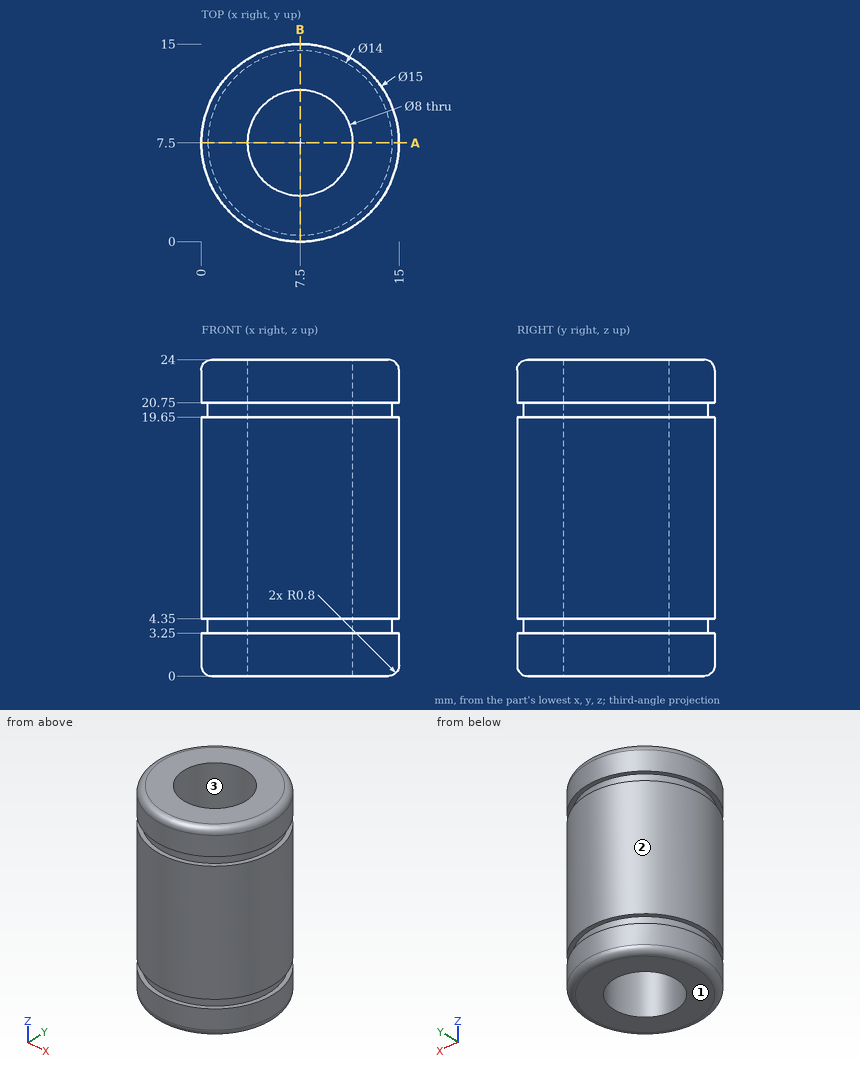
Geometry check sheet. Reference: drawing and pictorial views, mm from the part's lowest x, y, z. Coordinates: 2 decimals unless noted, no trailing zeros. Order: outer loops, then holes, each group sorted by start corner. A loop starts at its lowest first (then second) coordinate and runs counter-clockwise, first axis right, second up. Notation, with made-up numbers: (32, -13.5) - (72, -13.5) arc R24 cw to (72, 21.5) - close; hole circle Ø6 at (45, 41.25). An arc over 180 degrees is marked (long way). Answer in a Markdown table with one row per item. Add a question column.
1) Material ranges on line 1 along Y through (x, z) = (7.5, 16.25); line 2 along Z through (x, y) = (3.5, 1.5); line 3 along X through (y, z) = (5, 6.75), recorded low to high. Write a range as [from, to].
2) Cross-section at A-A, the plane y = 7.5. Record the cut outline in (x, z).
3) Gauge pin test, flat ends, axial feed: P1, Ø2, axis at y = 13, z = 9.5, coming from the +X side; P2, Ø2, axis at x = 5, z = 3.5, coming from the +Y side; P3, Ø1, axis at x = 13.5, z = 6, coming from the +Y side; P4, Ø4.5, axis at x = 8, y = 8.5, coming from the -Z side. Record the tip position at first contact, or that the pin passes through.
4) Release check for a two-part mould opening along X. For the marked faces 1, 2 and 3 record: +X half, -X half, draft (parallel to the pull), parting line (faces both ways), or undercut.
Check result:
| question | item | result |
|---|---|---|
| 1 | line 1 | y = [0, 3.5], [11.5, 15] |
| 1 | line 2 | z = [0.18, 3.25], [4.35, 19.65], [20.75, 23.82] |
| 1 | line 3 | x = [0.43, 4.38], [10.62, 14.57] |
| 2 | outline | (0, 0.8) arc R0.8 ccw to (0.8, 0) - (3.5, 0) - (3.5, 24) - (0.8, 24) arc R0.8 ccw to (0, 23.2) - (0, 20.75) - (0.5, 20.75) - (0.5, 19.65) - (0, 19.65) - (0, 4.35) - (0.5, 4.35) - (0.5, 3.25) - (0, 3.25) - close; (11.5, 0) - (14.2, 0) arc R0.8 ccw to (15, 0.8) - (15, 3.25) - (14.5, 3.25) - (14.5, 4.35) - (15, 4.35) - (15, 19.65) - (14.5, 19.65) - (14.5, 20.75) - (15, 20.75) - (15, 23.2) arc R0.8 ccw to (14.2, 24) - (11.5, 24) - close |
| 3 | P1 | stops at x = 13.5 |
| 3 | P2 | stops at y = 14.84 |
| 3 | P3 | stops at y = 12.6 |
| 3 | P4 | passes through |
| 4 | face 1 | draft |
| 4 | face 2 | parting line |
| 4 | face 3 | undercut |
